Source: CAD feature listing. Evaluate the final solid. Frame: model axes, mm. Face numbers are marked on the shaded views. A direction names the side the tool comes from. Round coordinates to 2 decimals unless told otherwise and drop trailing zeros. Loops run counter-clockwise (first coordinate to the right, second up) from the corner with the lowest first, then second, coordinate; pieces in that order, holes last. Notation, with made-up numbers: (50.5, 41) -> (91.5, 41) arc R24 ccw to (91.5, 54) -> close; hole circle Ø1 at (-36, -28.75). An arc over 180 degrees is marked (long way). Put each result on its own line as item: value. Start each with the question number.
1. Cut plane C-C (y = 4). Return the cut outline in (x, z).
2. Material intervals for L1, parallel to Z at x = -7, y = -53; L2, parallel to Y at x = -11, z = 49; L3, parallel to Z at x = 0, y = -60.75, sorted ascending.
3. Cut plane B-B (x = 0). Return the cut outline in (y, z), then the cut area to 3 significant figures.
4. Draft query along X for the marked faces 1, 2, 3 and 4. Return one class per face: pulls with the +X half, pulls with the -X half, needs draft (parallel to the pull), parting line crosses it, or undercut.
5. Set-up query: the marked faces 5, 6, 7 and 8. Return all of +Z, -Z, +X, -X, +Y, -Y with unobstructed straight access to the full face (end or side cutting, diameter ignored); none if empty.
6. Cut plane A-A (z = 31). Return the cut outline in (x, y).
7. Contact query for flat-ended pins moving along their axis: pin 1 (4 mm diameter, centred on x = -16.5, y = -14.5, fed in from +Z); pin 2 (12 mm diameter, centred on y = -0.5, z = 25.5, fed in from -X); pin 3 (6.5 mm diameter, centred on x = -2, y = -55, fed in from -Z). Output: stop coordinate, or through.
8. Cut plane D-D (y = -28). Return the cut outline in (x, z), then the cut area to 3 significant figures.
```python
from build123d import *

# Parameters (mm, degrees)
F0_R     = 20
F1_DEPTH = 25
F3_DEPTH = 15
F4_R     = 7.386866
F5_DEPTH = 125
F6_R     = 8.5
F7_DEPTH = 25


with BuildPart() as f1:
    # F0 (on Front) → F1 (new body)
    with BuildSketch(Plane.XZ):
        with Locations((-2.691098, 9.489658)):
            Circle(F0_R)
    extrude(amount=F1_DEPTH)

    # F2 (on face) → F3 (join)
    with BuildSketch(Plane(origin=(0, 0, 0), x_dir=(-1, 0, 0), z_dir=(0, 1, 0))):
        with BuildLine():
            ThreePointArc((-16.315418, 5.920409), (-11.92202, -4.686193), (-1.315418, -9.079591))
            Line((-1.315418, -9.079591), (6.684582, -9.079591))
            ThreePointArc((6.684582, -9.079591), (17.291184, -4.686193), (21.684582, 5.920409))
            Line((21.684582, 5.920409), (21.684582, 53.920409))
            ThreePointArc((21.684582, 53.920409), (17.291184, 64.527011), (6.684582, 68.920409))
            Line((6.684582, 68.920409), (-1.315418, 68.920409))
            ThreePointArc((-1.315418, 68.920409), (-11.92202, 64.527011), (-16.315418, 53.920409))
            Line((-16.315418, 53.920409), (-16.315418, 5.920409))
        make_face()
    extrude(amount=F3_DEPTH)

    # F4 (on face) → F5 (cut)
    with BuildSketch(Plane(origin=(0, 15, 0), x_dir=(-1, 0, 0), z_dir=(0, 1, 0))):
        with Locations((2.691099, 6.940198)):
            Circle(F4_R)
    extrude(amount=-F5_DEPTH, mode=Mode.SUBTRACT)

    # F6 (on face) → F7 (cut)
    with BuildSketch(Plane(origin=(0, 15, 0), x_dir=(-1, 0, 0), z_dir=(0, 1, 0))):
        with Locations((0, 53.43134)):
            Circle(F6_R)
    extrude(amount=-F7_DEPTH, mode=Mode.SUBTRACT)

    # F8: F1 across face


with BuildPart() as f1_1:
    add(f1.part)
    add(f1.part.mirror(Plane(origin=(-2.691098, -25, 9.892378), x_dir=(1, 0, 0), z_dir=(0, -1, 0))))


solid = f1_1.part
```
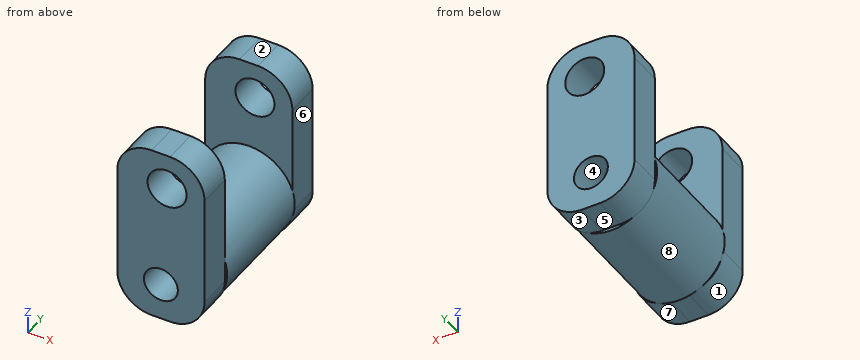
Solution:
1. outline: (-21.68, 5.92) arc R15 ccw to (-6.68, -9.08) -> (1.32, -9.08) arc R15 ccw to (16.32, 5.92) -> (16.32, 53.92) arc R15 ccw to (1.32, 68.92) -> (-6.68, 68.92) arc R15 ccw to (-21.68, 53.92) -> close; hole circle Ø14.77 at (-2.69, 6.94); hole circle Ø17 at (0, 53.43)
2. L1: z = -9.08 to 0.94, 12.94 to 48.61, 58.25 to 68.92
2. L2: y = -65 to -50, 0 to 15
2. L3: z = -9.08 to 0.06, 13.82 to 44.93, 61.93 to 68.92
3. outline: (-65, -9.08) -> (-50, -9.08) -> (-50, -10.33) -> (0, -10.33) -> (0, -9.08) -> (15, -9.08) -> (15, 0.06) -> (-65, 0.06) -> close; (-65, 13.82) -> (15, 13.82) -> (15, 44.93) -> (0, 44.93) -> (0, 29.31) -> (-50, 29.31) -> (-50, 44.93) -> (-65, 44.93) -> close; (-65, 61.93) -> (-50, 61.93) -> (-50, 68.92) -> (-65, 68.92) -> close; (0, 61.93) -> (15, 61.93) -> (15, 68.92) -> (0, 68.92) -> close
3. area: 2,710 mm^2
4. face 1: pulls with the -X half
4. face 2: needs draft
4. face 3: pulls with the +X half
4. face 4: undercut
5. face 5: -Z, +X, -X, +Y
5. face 6: +Z, -Z, +X, +Y
5. face 7: -Z, +X, -Y
5. face 8: none
6. outline: (-21.68, -65) -> (16.32, -65) -> (16.32, -50) -> (-21.68, -50) -> close; (-21.68, 0) -> (16.32, 0) -> (16.32, 15) -> (-21.68, 15) -> close
7. pin 1: stops at z = 25.63
7. pin 2: stops at x = -21.68
7. pin 3: stops at z = -9.08
8. outline: circle Ø40 at (-2.69, 9.49); hole circle Ø14.77 at (-2.69, 6.94)
8. area: 1,090 mm^2
